from build123d import *

# Parameters (mm, degrees)
SKETCH_1_W          = 27.399999997
SKETCH_1_H          = 4
EXTRUDE_1_DEPTH     = 3
SKETCH_1_3_W        = 27.399999997
SKETCH_1_3_H        = 4
EXTRUDE_2_DEPTH     = 11
SKETCH_1_4_W        = 27.399999997
SKETCH_1_4_H        = 4
EXTRUDE_3_DEPTH     = 8
SKETCH_2_R          = 1.5
CUT_EXTRUDE_1_DEPTH = 6.5
FILLET_1_R          = 4
EXTRUDE_4_DEPTH     = 19
SKETCH_6_W          = 32.257266432
SKETCH_6_H          = 23.708854684
CUT_EXTRUDE_2_DEPTH = 21
SKETCH_7_W          = 8
SKETCH_7_H          = 4
EXTRUDE_5_DEPTH     = 5
SKETCH_8_W          = 8
SKETCH_8_H          = 4
EXTRUDE_6_DEPTH     = 5
SKETCH_9_W          = 47.208598766
SKETCH_9_H          = 30.653056474
CUT_EXTRUDE_3_DEPTH = 18
FILLET_2_R          = 5


with BuildPart() as part:
    # 草图1 → 凸台-拉伸1 (new body)
    with BuildSketch(Plane.XY):
        with BuildLine():
            ThreePointArc((-0.337371922, -1.853501365), (-0.488220409, -1.87454383), (-0.640366957, -1.881577989))
            Line((-0.640366957, -1.881577989), (-1.640366957, -1.881577989))
            Line((-1.640366957, -1.881577989), (-1.640366957, -2.881577989))
            Line((-1.640366957, -2.881577989), (25.75963304, -2.881577989))
            Line((25.75963304, -2.881577989), (25.75963304, -1.88157799))
            Line((25.75963304, -1.88157799), (24.75963304, -1.88157799))
            ThreePointArc((24.75963304, -1.88157799), (24.607486492, -1.87454383), (24.456638005, -1.853501365))
            ThreePointArc((24.456638005, -1.853501365), (23.608703525, -1.413476758), (23.147062635, -0.577114262))
            ThreePointArc((23.147062635, -0.577114262), (22.880535784, 0.365382964), (22.493851477, 1.265278974))
            ThreePointArc((22.493851477, 1.265278974), (21.584633042, 1.287629087), (20.675414607, 1.265278974))
            ThreePointArc((20.675414607, 1.265278974), (20.288730299, 0.365382964), (20.022203448, -0.577114261))
            ThreePointArc((20.022203448, -0.577114261), (19.560562558, -1.413476758), (18.712628078, -1.853501365))
            ThreePointArc((18.712628078, -1.853501365), (18.409633042, -1.88157799), (18.106638005, -1.853501365))
            ThreePointArc((18.106638005, -1.853501365), (17.258703525, -1.413476758), (16.797062635, -0.577114262))
            ThreePointArc((16.797062635, -0.577114262), (16.530535784, 0.365382964), (16.143851477, 1.265278974))
            ThreePointArc((16.143851477, 1.265278974), (15.234633042, 1.287629087), (14.325414607, 1.265278974))
            ThreePointArc((14.325414607, 1.265278974), (13.938730299, 0.365382964), (13.672203448, -0.577114261))
            ThreePointArc((13.672203448, -0.577114261), (13.210562558, -1.413476758), (12.362628078, -1.853501365))
            ThreePointArc((12.362628078, -1.853501365), (12.059633042, -1.88157799), (11.756638005, -1.853501365))
            ThreePointArc((11.756638005, -1.853501365), (10.908703525, -1.413476758), (10.447062635, -0.577114262))
            ThreePointArc((10.447062635, -0.577114262), (10.180535784, 0.365382964), (9.793851477, 1.265278974))
            ThreePointArc((9.793851477, 1.265278974), (8.884633042, 1.287629087), (7.975414607, 1.265278974))
            ThreePointArc((7.975414607, 1.265278974), (7.588730299, 0.365382964), (7.322203448, -0.577114261))
            ThreePointArc((7.322203448, -0.577114261), (6.860562558, -1.413476758), (6.012628078, -1.853501365))
            ThreePointArc((6.012628078, -1.853501365), (5.709633042, -1.88157799), (5.406638005, -1.853501365))
            ThreePointArc((5.406638005, -1.853501365), (4.558703525, -1.413476758), (4.097062635, -0.577114262))
            ThreePointArc((4.097062635, -0.577114262), (3.830535784, 0.365382964), (3.443851477, 1.265278974))
            ThreePointArc((3.443851477, 1.265278974), (2.534633042, 1.287629087), (1.625414607, 1.265278974))
            ThreePointArc((1.625414607, 1.265278974), (1.238730299, 0.365382964), (0.972203448, -0.577114261))
            ThreePointArc((0.972203448, -0.577114261), (0.510562558, -1.413476758), (-0.337371922, -1.853501365))
        make_face()
        with Locations((12.059633041, -4.881577989)):
            Rectangle(SKETCH_1_W, SKETCH_1_H)
    extrude(amount=EXTRUDE_1_DEPTH)

    # 草图1<3> → 凸台-拉伸2 (add)
    with BuildSketch(Plane.XY):
        with Locations((12.059633041, -4.881577989)):
            Rectangle(SKETCH_1_3_W, SKETCH_1_3_H)
    extrude(amount=EXTRUDE_2_DEPTH)

    # 草图1<4> → 凸台-拉伸3 (add)
    with BuildSketch(Plane.XY):
        with Locations((12.059633041, -4.881577989)):
            Rectangle(SKETCH_1_4_W, SKETCH_1_4_H)
    extrude(amount=-EXTRUDE_3_DEPTH)

    # 草图2 → 切除-拉伸1 (cut)
    with BuildSketch(Plane(origin=(0, -2.881577989, 0), x_dir=(1, 0, 0), z_dir=(0, 1, 0))):
        with Locations(Location((2.059633042, 4.5, 0), (0, 0, 270))):
            Circle(SKETCH_2_R)
        with Locations(Location((22.059633042, 4.5, 0), (0, 0, 270))):
            Circle(SKETCH_2_R)
        with Locations(Location((22.059633042, -7.5, 0), (0, 0, 270))):
            Circle(SKETCH_2_R)
        with Locations(Location((2.059633042, -7.5, 0), (0, 0, 270))):
            Circle(SKETCH_2_R)
    extrude(amount=-CUT_EXTRUDE_1_DEPTH, mode=Mode.SUBTRACT)

    # 圆角1
    fillet_1_edges = [part.edges().sort_by_distance(p)[0] for p in [
        (-1.640366957, -4.881577989, 11),
        (-1.640366957, -4.881577989, -8),
    ]]
    fillet(fillet_1_edges, radius=FILLET_1_R)

    # 草图4 → 凸台-拉伸4 (add)
    with BuildSketch(Plane(origin=(0, 0, -8), x_dir=(-1, 0, 0), z_dir=(0, 0, -1))):
        with BuildLine():
            Line((-11.559633042, -6.881577989), (-16.559633042, -6.881577989))
            Line((-16.559633042, -6.881577989), (-16.559633042, -12.881577989))
            ThreePointArc((-16.559633042, -12.881577989), (-11.842889335, -20.796987993), (-2.636585146, -20.415740147))
            Line((-2.636585146, -20.415740147), (-2.636585146, -19.612245623))
            ThreePointArc((-2.636585146, -19.612245623), (-8.775001634, -18.470018526), (-11.559633042, -12.881577989))
            Line((-11.559633042, -12.881577989), (-11.559633042, -6.881577989))
        make_face()
    extrude(amount=-EXTRUDE_4_DEPTH)

    # 草图6 → 切除-拉伸2 (cut)
    with BuildSketch(Plane.XZ.offset(6.881577989)):
        with Locations((13.405653676, 0.508195322)):
            Rectangle(SKETCH_6_W, SKETCH_6_H)
    extrude(amount=CUT_EXTRUDE_2_DEPTH, mode=Mode.SUBTRACT)

    # 草图7 → 凸台-拉伸5 (add)
    with BuildSketch(Plane.XY.offset(11)):
        with Locations((21.75963304, -4.881577989)):
            Rectangle(SKETCH_7_W, SKETCH_7_H)
    extrude(amount=EXTRUDE_5_DEPTH)

    # 草图8 → 凸台-拉伸6 (add)
    with BuildSketch(Plane(origin=(0, 0, -8), x_dir=(-1, 0, 0), z_dir=(0, 0, -1))):
        with Locations((-21.75963304, -4.881577989)):
            Rectangle(SKETCH_8_W, SKETCH_8_H)
    extrude(amount=EXTRUDE_6_DEPTH)

    # 草图9 → 切除-拉伸3 (cut)
    with BuildSketch(Plane(origin=(0, -2.881577989, 0), x_dir=(1, 0, 0), z_dir=(0, 1, 0))):
        with Locations((10.799915409, -0.879700666)):
            Rectangle(SKETCH_9_W, SKETCH_9_H)
    extrude(amount=CUT_EXTRUDE_3_DEPTH, mode=Mode.SUBTRACT)

    # 圆角2
    fillet_2_edges = [part.edges().sort_by_distance(p)[0] for p in [
        (17.75963304, -4.881577989, 11),
        (17.75963304, -4.881577989, -8),
    ]]
    fillet(fillet_2_edges, radius=FILLET_2_R - 0.0001)  # a hair under: the kernel refuses the full size


solid = part.part
Input: part model. Units: mm. Frame: model coordinates. A direction names the side the tool comes from. Round coordinates to 2 decimals unless told otherwise and drop trailing zeros. Order: outer loops, then holes, each group sorted by start corner. A loop starts at its lowest first (then second) coordinate and runs counter-clockwise, first axis right, second up.
1. Cut plane B-B, the plane z = 7.5. Output: boundary loops of the cut face in (x, y), then the cut area to 3 significant figures.
The answers:
outline: (-1.61, -6.88) - (0.56, -6.88) - (0.56, -2.88) - (-1.61, -2.88) - close; (3.56, -6.88) - (20.56, -6.88) - (20.56, -2.88) - (3.56, -2.88) - close; (23.56, -6.88) - (25.76, -6.88) - (25.76, -2.88) - (23.56, -2.88) - close
area: 85.5 mm2
2. Cut plane C-C, the plane y = -6.5. State how many separate pieces and enclosed holes the cut face has, then the cut area to 3 significant figures.
The answers:
separate pieces: 1
enclosed holes: 4
area: 576 mm2
3. Mould query, pull axis Z, two halves, no side actions, for faces 1 (the face through (15, -2.882, 1)), 2 (the face through (20.595, -4.854, 7.175)), 3 (the face through (-0.5, -4.854, 9.797)). Classes: released by +Z, released by -Z, zero draft, split by the parting line, or undercut.
The answers:
face 1: zero draft
face 2: undercut
face 3: released by +Z
4. Cut plane D-D, the plane x = 7.5. Output: boundary loops of the cut face in (y, z), then the cut area to 3 significant figures.
The answers:
outline: (-6.88, -8) - (-2.88, -8) - (-2.88, 11) - (-6.88, 11) - close
area: 76.0 mm2
5. Material intervals for line 1 (X direction, y = -5.7, z = -4.5); line 2 (Z direction, x = 20.75, y = -6.6); line 3 (Z direction, x = 22.75, y = -5.4), sorted ascending.
The answers:
line 1: x = -1.61 to 0.56, 3.56 to 20.56, 23.56 to 25.76
line 2: z = -13 to -5.23, -3.77 to 6.77, 8.23 to 16
line 3: z = -13 to -5.83, -3.17 to 6.17, 8.83 to 16
6. Cut plane A-A, the plane x = 22.5. Output: boundary loops of the cut face in (y, z), then the cut area to 3 significant figures.
The answers:
outline: (-6.88, -13) - (-2.88, -13) - (-2.88, -5.93) - (-6.88, -5.93) - close; (-6.88, -3.07) - (-2.88, -3.07) - (-2.88, 6.07) - (-6.88, 6.07) - close; (-6.88, 8.93) - (-2.88, 8.93) - (-2.88, 16) - (-6.88, 16) - close
area: 93.1 mm2
7. Pin query (flat end, axial travel): P1, Ø1.2, axis at x = 9, y = -5, coming from the -Z side; P2, Ø2.5, axis at x = 2.06, z = 7.5, coming from the +Y side; P3, Ø5, axis at x = 22.06, z = -4.5, coming from the -Y side. Return the tip coordinate at first contact, or that it passes through.
The answers:
P1: stops at z = -8
P2: passes through
P3: stops at y = -6.88
8. Set-up query: faces 4 (the face through (20.595, -4.854, -4.825)), 5 (the face through (7, -5, -8)), 6 (the face through (7, -5, 11)). Return all of +Z, -Z, +X, -X, +Y, -Y with unobstructed straight access to the full face (end or side cutting, diameter ignored); none if empty.
The answers:
face 4: +Y, -Y
face 5: -Z, -X, +Y, -Y
face 6: +Z, -X, +Y, -Y
